from build123d import *

# Parameters (mm, degrees)
F0_W      = 93.98
F0_H      = 152.4
F1_DEPTH  = 12.7
F2_W      = 82.55
F2_H      = 57.15
F3_DEPTH  = 10.16
F5_W      = 12.7
F5_H      = 12.7
F6_DEPTH  = 6.1722
F7_R      = 1.524
F8_DEPTH  = 6.1722
F9_W      = 17.145
F9_H      = 50.8
F10_DEPTH = 10.16


with BuildPart() as f1:
    # F0 (on Top) → F1 (new body)
    with BuildSketch(Plane.XY):
        with Locations((46.99, 76.2)):
            Rectangle(F0_W, F0_H)
    extrude(amount=-F1_DEPTH)

    # F2 (on Top) → F3 (cut)
    with BuildSketch(Plane.XY):
        with Locations((46.99, 111.125)):
            Rectangle(F2_W, F2_H)
    extrude(amount=-F3_DEPTH, mode=Mode.SUBTRACT)

    # F5 (on face) → F6 (join)
    with BuildSketch(Plane.XY.offset(-10.16)):
        with Locations((12.065, 133.35)):
            Rectangle(F5_W, F5_H)
        with Locations((81.915, 133.35)):
            Rectangle(F5_W, F5_H)
        with Locations((12.065, 88.9)):
            Rectangle(F5_W, F5_H)
        with Locations((81.915, 88.9)):
            Rectangle(F5_W, F5_H)
    extrude(amount=F6_DEPTH)

    # F7 (on face) → F8 (cut)
    with BuildSketch(Plane.XY.offset(-3.9878)):
        with Locations((12.192, 133.223)):
            Circle(F7_R)
        with Locations((81.788, 133.223)):
            Circle(F7_R)
        with Locations((12.192, 89.027)):
            Circle(F7_R)
        with Locations((81.788, 89.027)):
            Circle(F7_R)
    extrude(amount=-F8_DEPTH, mode=Mode.SUBTRACT)

    # F9 (on face) → F10 (cut)
    with BuildSketch(Plane.XY):
        with Locations((46.99, 63.5)):
            Rectangle(F9_W, F9_H)
    extrude(amount=-F10_DEPTH, mode=Mode.SUBTRACT)


solid = f1.part
The listing builds one solid part. Answer for the finished solid, in the listing's coordinates (mm). A direction names the side the tool comes from. Coordinates: 2 decimals unless noted, no trailing zeros. Loops run counter-clockwise (first coordinate to the right, second up) from the corner with the lowest first, then second, coordinate; pieces in that order, holes last. Notation, with made-up numbers: (50, -35) -> (56, -35) arc R27 ccw to (56, -13) -> close; hole circle Ø6 at (-32.75, 89.5). An arc over 180 degrees is marked (long way). Answer in a Markdown table with one row per item. Add a question column.
1. For faces 4 (the flat face through (18.415, 89, -7)), 5 (the flat face through (46, 0, -6)), determine the directions among +Z, -Z, +X, -X, +Y, -Y from which every point of the face is accessible in a straight line to the end or side of a thin tool.
2. Flat-ended cylindrical pins translate along their axes: P1, Ø2.5, axis at x = 12.192, y = 133.223, coming from the +Z side; P2, Ø10, axis at x = 21.5, y = 97.5, coming from the +Z side. Find the tip coordinate at first contact, or state that the pin passes through.
3. The part is cut by section C-C, the plane x = 46.5. Write down the section's boundary in (y, z), then the cut area to 3 significant figures.
4. The part is cut by section A-A, the plane y = 123. Write down the section's boundary in (x, z) (3 decimals).
5. Determine the mould class of faces 1 (the flat face through (46, 152.4, -6)), 2 (the flat face through (0, 75, -6)), 3 (the flat face through (83.2, 90.4, -3.988)) for opening direction Y: +Y half, -Y half, draft (parallel to the pull), parting line (faces both ways), or undercut.
6. Consider line 1 (Y direction, x = 22, z = -2.25); line 2 (X direction, y = 102, z = -7.75) (3 decimals); line 3 (Y direction, x = 86, z = -4.25). Determine where each line is inside the solid, lowest interval first. Write a range as [from, to].
Answer below:
| question | item | result |
|---|---|---|
| 1 | face 4 | +Z |
| 1 | face 5 | +Z, -Z, +X, -X, -Y |
| 2 | P1 | z = -10.16 |
| 2 | P2 | z = -3.99 |
| 3 | outline | (0, -12.7) -> (152.4, -12.7) -> (152.4, 0) -> (139.7, 0) -> (139.7, -10.16) -> (38.1, -10.16) -> (38.1, 0) -> (0, 0) -> close |
| 3 | area | 903 mm2 |
| 4 | outline | (0, -12.7) -> (93.98, -12.7) -> (93.98, 0) -> (88.265, 0) -> (88.265, -10.16) -> (5.715, -10.16) -> (5.715, 0) -> (0, 0) -> close |
| 5 | face 1 | +Y half |
| 5 | face 2 | draft |
| 5 | face 3 | undercut |
| 6 | line 1 | [0, 82.55], [139.7, 152.4] |
| 6 | line 2 | [0, 5.715], [88.265, 93.98] |
| 6 | line 3 | [0, 95.25], [127, 152.4] |
